from build123d import *

# Parameters (mm, degrees)
F0_W     = 65
F0_H     = 50
F0_W_2   = 45
F0_H_2   = 6.7
F1_DEPTH = 8
F2_R     = 6
F2_R_2   = 3.6
F2_R_3   = 5
F2_R_4   = 2.55
F3_DEPTH = 4
F4_W     = 5.5
F4_H     = 6.7
F5_DEPTH = 3
F6_R     = 5
F8_DEPTH = 25


with BuildPart() as f1:
    # F0 (on Front) → F1 (new body)
    with BuildSketch(Plane.XZ):
        Rectangle(F0_W, F0_H)
        with BuildLine():
            ThreePointArc((-24.5, 12.35), (-27.0455844123, 18.4955844123), (-20.9, 15.95))
            Line((-20.9, 15.95), (20.9, 15.95))
            ThreePointArc((20.9, 15.95), (24.5, 19.55), (28.1, 15.95))
            ThreePointArc((28.1, 15.95), (27.0455844123, 13.4044155877), (24.5, 12.35))
            Line((24.5, 12.35), (24.5, 3.35))
            Line((24.5, 3.35), (27, 3.35))
            Line((27, 3.35), (27, -3.35))
            Line((27, -3.35), (24.5, -3.35))
            Line((24.5, -3.35), (24.5, -13.4))
            ThreePointArc((24.5, -13.4), (26.303122292, -14.146877708), (27.05, -15.95))
            ThreePointArc((27.05, -15.95), (24.5, -18.5), (21.95, -15.95))
            Line((21.95, -15.95), (-21.95, -15.95))
            ThreePointArc((-21.95, -15.95), (-26.303122292, -17.753122292), (-24.5, -13.4))
            Line((-24.5, -13.4), (-24.5, -3.35))
            Line((-24.5, -3.35), (-27, -3.35))
            Line((-27, -3.35), (-27, 3.35))
            Line((-27, 3.35), (-24.5, 3.35))
            Line((-24.5, 3.35), (-24.5, 12.35))
        make_face(mode=Mode.SUBTRACT)
        with BuildLine():
            Line((20.9, 15.95), (-20.9, 15.95))
            ThreePointArc((-20.9, 15.95), (-21.9544155877, 13.4044155877), (-24.5, 12.35))
            Line((-24.5, 12.35), (-24.5, 3.35))
            Line((-24.5, 3.35), (-22.5, 3.35))
            Line((-22.5, 3.35), (22.5, 3.35))
            Line((22.5, 3.35), (24.5, 3.35))
            Line((24.5, 3.35), (24.5, 12.35))
            ThreePointArc((24.5, 12.35), (21.9544155877, 13.4044155877), (20.9, 15.95))
        make_face()
        with BuildLine():
            Line((-22.5, -3.35), (-24.5, -3.35))
            Line((-24.5, -3.35), (-24.5, -13.4))
            ThreePointArc((-24.5, -13.4), (-22.696877708, -14.146877708), (-21.95, -15.95))
            Line((-21.95, -15.95), (21.95, -15.95))
            ThreePointArc((21.95, -15.95), (22.696877708, -14.146877708), (24.5, -13.4))
            Line((24.5, -13.4), (24.5, -3.35))
            Line((24.5, -3.35), (22.5, -3.35))
            Line((22.5, -3.35), (-22.5, -3.35))
        make_face()
        Rectangle(F0_W_2, F0_H_2)
    extrude(amount=F1_DEPTH)

    # F2 (on face) → F3 (cut)
    with BuildSketch(Plane.XZ.offset(8)):
        with Locations((24.5, 15.95)):
            Circle(F2_R)
        with Locations((24.5, 15.95)):
            Circle(F2_R_2, mode=Mode.SUBTRACT)
        with Locations((-24.5, 15.95)):
            Circle(F2_R)
        with Locations((-24.5, 15.95)):
            Circle(F2_R_2, mode=Mode.SUBTRACT)
        with Locations((-24.5, -15.95)):
            Circle(F2_R_3)
        with Locations((-24.5, -15.95)):
            Circle(F2_R_4, mode=Mode.SUBTRACT)
        with Locations((24.5, -15.95)):
            Circle(F2_R_3)
        with Locations((24.5, -15.95)):
            Circle(F2_R_4, mode=Mode.SUBTRACT)
    extrude(amount=-F3_DEPTH, mode=Mode.SUBTRACT)

    # F4 (on face) → F5 (cut)
    with BuildSketch(Plane.XZ.offset(8)):
        with Locations((29.75, 0)):
            Rectangle(F4_W, F4_H)
        with Locations((-29.75, 0)):
            Rectangle(F4_W, F4_H)
    extrude(amount=-F5_DEPTH, mode=Mode.SUBTRACT)

    # F6
    f6_edges = [f1.edges().sort_by_distance(p)[0] for p in [
        (-32.5, -4, 25),
        (32.5, -4, 25),
        (32.5, -4, -25),
        (-32.5, -4, -25),
    ]]
    fillet(f6_edges, radius=F6_R)

    # F7 (on face) → F8 (cut)
    with BuildSketch(Plane.XZ.offset(8)):
        with BuildLine():
            Line((-15.5, 13.95), (-15.5, 15.5))
            Line((-15.5, 15.5), (-13.95, 15.5))
            ThreePointArc((-13.95, 15.5), (-16.5960155108, 16.5960155108), (-15.5, 13.95))
        make_face()
        with BuildLine():
            Line((-13.95, 15.5), (-15.5, 15.5))
            Line((-15.5, 15.5), (-15.5, 13.95))
            ThreePointArc((-15.5, 13.95), (-14.4039844892, 14.4039844892), (-13.95, 15.5))
        make_face()
        with BuildLine():
            ThreePointArc((-13.95, -15.5), (-14.4039844892, -14.4039844892), (-15.5, -13.95))
            Line((-15.5, -13.95), (-15.5, -15.5))
            Line((-15.5, -15.5), (-13.95, -15.5))
        make_face()
        with BuildLine():
            Line((-15.5, -15.5), (-15.5, -13.95))
            ThreePointArc((-15.5, -13.95), (-16.5960155108, -16.5960155108), (-13.95, -15.5))
            Line((-13.95, -15.5), (-15.5, -15.5))
        make_face()
        with BuildLine():
            Line((15.5, -15.5), (15.5, -13.95))
            ThreePointArc((15.5, -13.95), (14.4039844892, -14.4039844892), (13.95, -15.5))
            Line((13.95, -15.5), (15.5, -15.5))
        make_face()
        with BuildLine():
            ThreePointArc((17.05, -15.5), (16.5960155108, -14.4039844892), (15.5, -13.95))
            Line((15.5, -13.95), (15.5, -15.5))
            Line((15.5, -15.5), (13.95, -15.5))
            ThreePointArc((13.95, -15.5), (15.5, -17.05), (17.05, -15.5))
        make_face()
        with BuildLine():
            Line((15.5, 15.5), (13.95, 15.5))
            ThreePointArc((13.95, 15.5), (14.4039844892, 14.4039844892), (15.5, 13.95))
            Line((15.5, 13.95), (15.5, 15.5))
        make_face()
        with BuildLine():
            ThreePointArc((17.05, 15.5), (15.5, 17.05), (13.95, 15.5))
            Line((13.95, 15.5), (15.5, 15.5))
            Line((15.5, 15.5), (15.5, 13.95))
            ThreePointArc((15.5, 13.95), (16.5960155108, 14.4039844892), (17.05, 15.5))
        make_face()
    extrude(amount=-F8_DEPTH, mode=Mode.SUBTRACT)


solid = f1.part
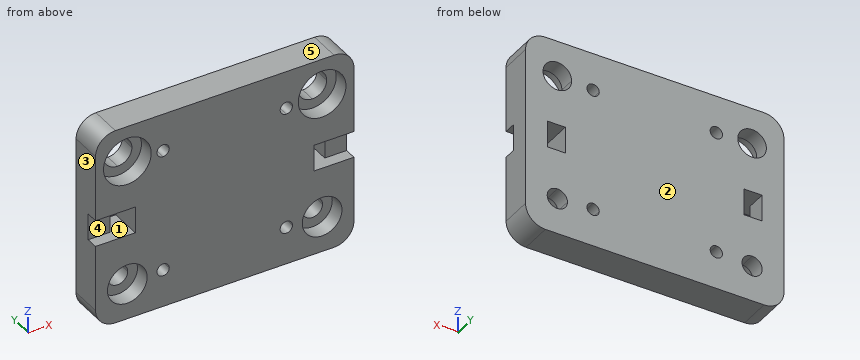
Geometry: final body of the model. Coordinates: model frame, mm. Face numbers are marked on the shaded views. A direction names the side the tool comes from. Coordinates: 2 decimals unless noted, no trailing zeros. Loops run counter-clockwise (first coordinate to the right, second up) from the corner with the lowest first, then second, coordinate; pieces in that order, holes last. Notation, with made-up numbers: (5, 16) - (16, 16) arc R23 cw to (16, 31) - close; hole circle Ø10 at (0.5, 78.5). An arc over 180 degrees is marked (long way). Put each result on its own line as item: value. Start each with the question number.
Q1. Line query: line 1 (X direction, y = -2.5, z = 0.5); line 2 (Z direction, x = -24.5, y = -1.6); line 3 (X direction, y = -7.25, z = 13). Output: solid intervals per line, ascending.
Q2. Cut plane A-A, the plane y = -6.75. Give the number of separate pieces and of enclosed holes in the cut face, and give its area (3 significant figures).
Q3. Cut plane C-C, the plane x = -26. Return loops of the section in (y, z).
Q4. Pin query (flat end, axial travel): pin 1 Ø12 at (x, z) = (-25.5, -16.5) entering from -Y; pin 2 Ø3 at (x, z) = (-31, 1) entering from -Y; pin 3 Ø6 at (x, z) = (22, 17) entering from -Y. Return the tip coordinate at first contact, or that it passes through.
Q5. Set-up query: the marked faces 1 and 2. Return all of +Z, -Z, +X, -X, +Y, -Y with unobstructed straight access to the full face (end or side cutting, diameter ignored); none if empty.
Q6. Pull-direction query (Z, two-part tool) for the marked faces 3, 4 and 5; classes: released by +Z, released by -Z, zero draft, split by the parting line, or undercut.
Filled sheet:
1. line 1: -32.5 to -27, -22.5 to 22.5, 27 to 32.5
1. line 2: -25 to -18.5, -13.4 to -3.35, 3.35 to 12.35, 19.55 to 25
1. line 3: -32.5 to -29.72, -19.28 to 19.28, 29.72 to 32.5
2. separate pieces: 1
2. enclosed holes: 8
2. area: 2,680 mm²
3. outline: (-8, -25) - (0, -25) - (0, -18.01) - (-4, -18.01) - (-4, -20.72) - (-8, -20.72) - close; (-8, -11.18) - (-4, -11.18) - (-4, -13.89) - (0, -13.89) - (0, -3.35) - (-8, -3.35) - close; (-8, 3.35) - (0, 3.35) - (0, 12.68) - (-4, 12.68) - (-4, 10.14) - (-8, 10.14) - close; (-8, 21.76) - (-4, 21.76) - (-4, 19.22) - (0, 19.22) - (0, 25) - (-8, 25) - close
4. pin 1: y = -8
4. pin 2: y = -5
4. pin 3: y = -4
5. face 1: -Y
5. face 2: +Z, -Z, +X, -X, +Y
6. face 3: zero draft
6. face 4: undercut
6. face 5: released by +Z
